Check sheet for the modelled part. Datum: model origin and axes. Units: mm. A direction names the side the tool comes from. Round coordinates to 2 decimals unless told otherwise and drop trailing zeros. Write each loop counter-clockwise with the first axis right and the second up, starting at its lowest first coordinate (ties: lowest second). Pieces come first, ordered by that corner, then holes. Notation, with made-up numbers: (55, -20.75) - (70, -20.75) arc R14 cw to (70, 2.25) - close; hole circle Ø2 at (86, 53). An arc over 180 degrees is marked (long way). Use one line per item in the form item = value. Start each with the question number.
1) Set-up check for faces 5 (the face through (7.73, 14.15, -26.24)), 6 (the face through (15, 0, -15)): record each of +Z, -Z, +X, -X, +Y, -Y from which the full face is reachable in a straight line by a thin tool's end or side.
2) Draft check along X on faces 1 (the face through (30, -0.4, -20.2)), 2 (the face through (15, -2.6, -17)), 3 (the face through (0, -0.4, -20.2)), 4 (the face through (15.168, -1.526, -7.824)). Enter one of: +X half, -X half, draft (parallel to the pull), parting line (faces both ways), or undercut.
3) Scan lines: probe 1 along Y at (x, z) = (17.75, -13); probe 2 along Z at (x, y) = (10.75, 16.25) (3 decimals). Record each from-to range of solid material in increasing order.
4) Gauge pin test, flat ends, axial feed: P1, Ø12.5, axis at x = 8, z = -8, coming from the +Y side; P2, Ø5, axis at x = 7.94, y = 12.58, coming from the +Z side (3 decimals); P3, Ø12, axis at y = 8, z = -4, coming from the +X side. Record the tip position at first contact, or that the pin passes through.
5) Section check D-D (z = -16). Record the boundary of the cut face in (x, y), then the cut area to 3 significant figures.
6) Section check C-C (y = 2.25). Record the boundary of the cut face in (x, z) (3 decimals).
from build123d import *

# Parameters (mm, degrees)
PROFILE_BOSS_EXTRUDE1_DEPTH      = 30
COLLARCUT_EXTRUDE1_DEPTH         = 46.78748337
COLLAR_CHAMFER2_SIZE             = 1.3
MOUNTINGHOLES_SKETCH3_R          = 1.5875
MOUNTINGHOLES_CUT_EXTRUDE2_DEPTH = 44.928655321


with BuildPart() as part:
    # Profile-Sketch1 → Profile-Boss-Extrude1 (new body)
    with BuildSketch(Plane(origin=(0, 0, 0), x_dir=(0, 0, -1), z_dir=(1, 0, 0))):
        Polygon((0, 0), (24.675, 0), (24.675, 20.515144), (27.85, 20.515144), (27.85, -2.6), (0, -2.6), align=None)
    extrude(amount=PROFILE_BOSS_EXTRUDE1_DEPTH)

    # CollarSketch2 → CollarCut-Extrude1 (cut, through all)
    with BuildSketch(Plane(origin=(0, 0, 0), x_dir=(1, 0, 0), z_dir=(0, 1, 0))):
        with BuildLine():
            Line((7.917627516, 0), (22.082372484, 0))
            ThreePointArc((22.082372484, 0), (15, 7.6), (7.917627516, 0))
        make_face()
    extrude(amount=-COLLARCUT_EXTRUDE1_DEPTH, mode=Mode.SUBTRACT)

    # Collar-Chamfer2
    collar_chamfer2_edges = [part.edges().sort_by_distance(p)[0] for p in [
        (15, -2.6, -7.6),
        (15, 0, -7.6),
    ]]
    chamfer(collar_chamfer2_edges, length=COLLAR_CHAMFER2_SIZE - 0.0001)  # a hair under: the kernel refuses the full size

    # MountingHoles-Sketch3 → MountingHoles-Cut-Extrude2 (cut, through all)
    with BuildSketch(Plane.XY.offset(-24.675)):
        with Locations((7.9375, 12.577644)):
            Circle(MOUNTINGHOLES_SKETCH3_R)
        with Locations((22.0625, 12.577644)):
            Circle(MOUNTINGHOLES_SKETCH3_R)
    extrude(amount=-MOUNTINGHOLES_CUT_EXTRUDE2_DEPTH, mode=Mode.SUBTRACT)


solid = part.part
Results are:
q1.face_5 = +Z, -Z
q1.face_6 = +Z, +X, -X, +Y
q2.face_1 = +X half
q2.face_2 = draft
q2.face_3 = -X half
q2.face_4 = undercut
q3.probe_1 = -2.6 to 0
q3.probe_2 = -27.85 to -24.675
q4.P1 = 0
q4.P2 = -24.675
q4.P3 = through
q5.outline = (0, -2.6) - (30, -2.6) - (30, 0) - (0, 0) - close
q5.area = 78.0 mm²
q6.outline = (0, -27.85) - (30, -27.85) - (30, -24.675) - (0, -24.675) - close
